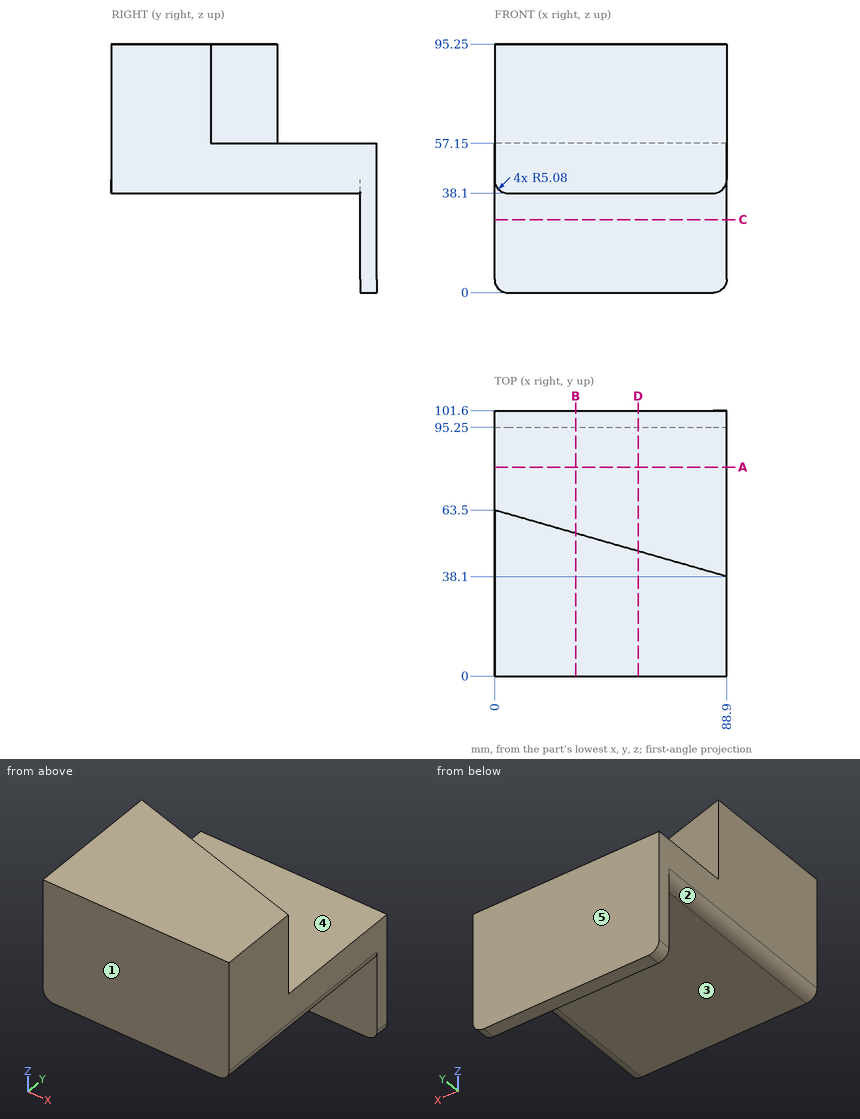
For this review, use the dimensioned drawing (mm, ordinates from the lowest corner) and the shaded views. A direction names the side the tool comes from. Round coordinates to 2 decimals unless told otherwise and drop trailing zeros. Order: outer loops, then holes, each group sorted by start corner. A loop starts at its lowest first (then second) coordinate and runs counter-clockwise, first axis right, second up. Notation, with made-up numbers: (72, 52) -> (102, 52) arc R8 ccw to (102, 57) -> close; hole circle Ø7 at (48.5, -30.5). An arc over 180 degrees is marked (long way). Put each result on its own line as item: value.
Q1. Machinability: for the marked faces 1, 2, 3, 4 and 5, which of the approach directions +Z, -Z, +X, -X, +Y, -Y give a long, thin tool a straight path to every point of the face, cutting with its end or side? Answer none if there is none.
Check result:
face 1: +Z, -Z, +X, -X, -Y
face 2: -Z, -X, -Y
face 3: -Z, +X, -X, -Y
face 4: +Z, +X, +Y
face 5: +Z, -Z, +X, -X, +Y
Q2. Add section A-A on y = 80. Write out the cut boundary in (x, z), plus the area to 3 significant figures.
Check result:
outline: (0, 43.18) arc R5.08 ccw to (5.08, 38.1) -> (83.82, 38.1) arc R5.08 ccw to (88.9, 43.18) -> (88.9, 57.15) -> (0, 57.15) -> close
area: 1,680 mm2
Q3. Add section D-D on x = 55. Write out the cut boundary in (y, z).
Check result:
outline: (0, 38.1) -> (95.25, 38.1) -> (95.25, 0) -> (101.6, 0) -> (101.6, 57.15) -> (47.79, 57.15) -> (47.79, 95.25) -> (0, 95.25) -> close
Q4. For probe 1 along Y at (x, z) = (14.5, 16); probe 2 along Z at (x, y) = (40.5, 89); probe 3 along Z at (x, y) = (27.5, 18), list the stretches that pass through material, from the lowest coordinate up. Write a range as [from, to].
Check result:
probe 1: [95.25, 101.6]
probe 2: [38.1, 57.15]
probe 3: [38.1, 95.25]
Q5. Add section C-C on z = 28. Write out the cut boundary in (x, y).
Check result:
outline: (0, 95.25) -> (88.9, 95.25) -> (88.9, 101.6) -> (0, 101.6) -> close
Q6. Add section B-B on x = 31. Write out the cut boundary in (y, z), plus the area to 3 significant figures.
Check result:
outline: (0, 38.1) -> (95.25, 38.1) -> (95.25, 0) -> (101.6, 0) -> (101.6, 57.15) -> (54.64, 57.15) -> (54.64, 95.25) -> (0, 95.25) -> close
area: 4,260 mm2
Q7. Insertion check: pin 1 Ø4 at (x, y) = (73.5, 54.5) entering from +Z; pin 2 Ø1.5 at (x, z) = (67, 70) entering from +Y; pin 3 Ø21.5 at (x, z) = (44.5, 14.5) entering from -Y. Each pin has a flat end and moves straight along its axis. Give the tip position at first contact, or say it passes through.
Check result:
pin 1: z = 57.15
pin 2: y = 44.57
pin 3: y = 95.25
